```python
from build123d import *

# Parameters (mm, degrees)
F0_W      = 200
F0_H      = 200
F1_DEPTH  = 19.05
F3_D      = 16
F4_W      = 12
F4_H      = 125
F5_DEPTH  = 75
F6_SIZE2  = 75
F6_SIZE   = 50
F9_DEPTH  = 19.05
F11_DEPTH = 500
F12_W     = 50
F12_H     = 5
F13_DEPTH = 90
F14_W     = 5
F14_H     = 80
F15_DEPTH = 70
F16_SIZE2 = 40
F16_SIZE  = 60
F18_DEPTH = 25
F19_W     = 65
F19_H     = 19.05
F20_DEPTH = 25
F21_R     = 10
F22_R     = 6
F23_DEPTH = 25


with BuildPart() as f1:
    # F0 (on Top) → F1 (new body)
    with BuildSketch(Plane.XY):
        Rectangle(F0_W, F0_H)
    extrude(amount=F1_DEPTH)

    # F3 (through all)
    with Locations(Plane.XY.offset(19.05)):
        with Locations((0, 80)):
            Hole(F3_D / 2)

    # F4 (on face) → F5 (join)
    with BuildSketch(Plane(origin=(0, 0, 0), x_dir=(1, 0, 0), z_dir=(0, 0, -1))):
        with Locations((79, 37.5)):
            Rectangle(F4_W, F4_H)
    extrude(amount=F5_DEPTH)

    # F6
    f6_edges = [f1.edges().sort_by_distance(p)[0] for p in [
        (79, 25, -75),
    ]]
    f6_side = f1.faces().sort_by_distance((79, 25, -37.5))[0]
    chamfer(f6_edges, length=F6_SIZE, length2=F6_SIZE2, reference=f6_side)

    # F7: F1 across plane


with BuildPart() as f1_1:
    add(f1.part)
    add(f1.part.mirror(Plane.YZ))

    # F8 (on face) → F9 (join)
    with BuildSketch(Plane.XZ.offset(100)):
        Polygon((100, -85.95), (100, 0), (85, 0), (85, -75), (73, -75), (73, 0), (-73, 0), (-73, -75), (-85, -75), (-85, 0), (-100, 0), (-100, -85.95), align=None)
        Polygon((100, 0), (100, 19.05), (-100, 19.05), (-100, 0), (-85, 0), (-85, -75), (-73, -75), (-73, 0), (73, 0), (73, -75), (85, -75), (85, 0), align=None)
    extrude(amount=F9_DEPTH)

    # F10 (on face) → F11 (cut)
    with BuildSketch(Plane.YZ.offset(85)):
        Polygon((-100, 0), (-100, -21.6502193362), (-68.8245669007, 0), align=None)
    extrude(amount=-F11_DEPTH, mode=Mode.SUBTRACT)

    # F12 (on face) → F13 (join)
    with BuildSketch(Plane(origin=(0, 0, 0), x_dir=(1, 0, 0), z_dir=(0, 0, -1))):
        with Locations((0, -62.5)):
            Rectangle(F12_W, F12_H)
    extrude(amount=F13_DEPTH)

    # F14 (on face) → F15 (join)
    with BuildSketch(Plane(origin=(0, 0, 0), x_dir=(1, 0, 0), z_dir=(0, 0, -1))):
        with Locations((0, -20)):
            Rectangle(F14_W, F14_H)
    extrude(amount=F15_DEPTH)

    # F16
    f16_edges = [f1_1.edges().sort_by_distance(p)[0] for p in [
        (0, -20, -70),
    ]]
    f16_side = f1_1.faces().sort_by_distance((0, 20, -70))[0]
    chamfer(f16_edges, length=F16_SIZE, length2=F16_SIZE2, reference=f16_side)

    # F17 (on face) → F18 (cut)
    with BuildSketch(Plane.YZ.offset(2.5)):
        Polygon((60, 0), (49.0511549105, 0), (60, -8.0538968956), align=None)
    extrude(amount=-F18_DEPTH, mode=Mode.SUBTRACT)

    # F19 (on face) → F20 (join)
    with BuildSketch(Plane(origin=(0, 100, 0), x_dir=(-1, 0, 0), z_dir=(0, 1, 0))):
        with Locations((67.5, 9.525)):
            Rectangle(F19_W, F19_H)
    extrude(amount=F20_DEPTH)

    # F21
    f21_edges = [f1_1.edges().sort_by_distance(p)[0] for p in [
        (-100, 125, 9.525),
        (-35, 125, 9.525),
        (-35, 100, 9.525),
    ]]
    fillet(f21_edges, radius=F21_R)

    # F22 (on face) → F23 (cut)
    with BuildSketch(Plane.XY.offset(19.05)):
        with Locations((-63.2194236771, 108.8713434036)):
            Circle(F22_R)
        with Locations((-68.7925902107, 70.10911874)):
            Circle(F22_R)
        with Locations((-52.5245954176, 34.4871789908)):
            Circle(F22_R)
        with Locations((-19.5804127005, 13.3152383338)):
            Circle(F22_R)
        with Locations((19.5804127005, 13.3152383338)):
            Circle(F22_R)
    extrude(amount=-F23_DEPTH, mode=Mode.SUBTRACT)


solid = f1_1.part
```
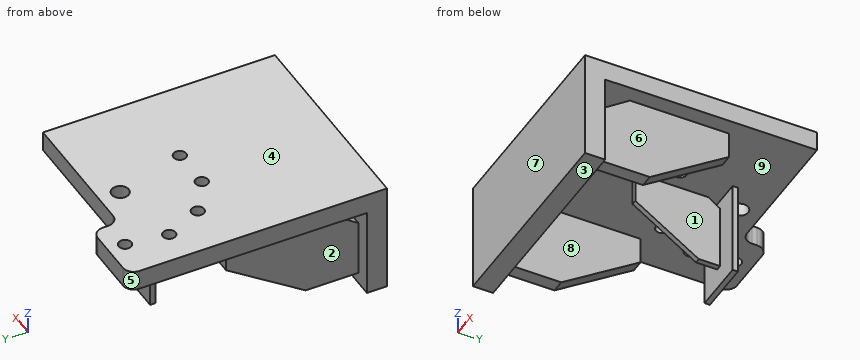
Model file for the job. Use its own axes, mm. Face numbers are marked on the shaded views. A direction names the side the tool comes from. Round coordinates to 2 decimals unless told otherwise and drop trailing zeros. Order: outer loops, then holes, each group sorted by start corner. A loop starts at its lowest first (then second) coordinate and runs counter-clockwise, first axis right, second up. Notation, with made-up numbers: (-8.75, -38.5) -> (11.25, -38.5) arc R14 ccw to (11.25, -15.5) -> close; hole circle Ø10 at (-37, -23.75). An arc over 180 degrees is marked (long way). Use one line per item in the form item = value.
Item 1: Cut at A-A, the plane z = -39.5. Write the cut outline in (x, y), and give its area (3 significant figures).
Returned:
outline = (-100, -119.05) -> (100, -119.05) -> (100, -100) -> (85, -100) -> (85, 3.25) -> (73, 3.25) -> (73, -100) -> (-73, -100) -> (-73, 3.25) -> (-85, 3.25) -> (-85, -100) -> (-100, -100) -> close; (-25, 60) -> (-2.5, 60) -> (-2.5, -5.75) -> (2.5, -5.75) -> (2.5, 60) -> (25, 60) -> (25, 65) -> (-25, 65) -> close
area = 6,870 mm^2
Item 2: Cut at B-B, the plane y = 80. Write the cut outline in (x, z), and give its area (3 significant figures).
Returned:
outline = (-100, 0) -> (-8, 0) -> (-8, 19.05) -> (-100, 19.05) -> close; (8, 0) -> (100, 0) -> (100, 19.05) -> (8, 19.05) -> close
area = 3,510 mm^2
Item 3: Tool access for the marked faces 1, 2, 3, 4 and 5: list every direction of +Z, -Z, +X, -X, +Y, -Y with a clear straight run to the whole face (end or side of a thin tool).
Returned:
face_1 = -Z
face_2 = -Z, -X, +Y
face_3 = -Z, +X, -X, -Y
face_4 = +Z, +X, -X, +Y, -Y
face_5 = +Z, -Z, -X, +Y
Item 4: Drill centre lines: line 1 (X direction, y = -87, z = -47); line 2 (Y direction, x = 3, z = -10); line 3 (Z direction, x = -5, y = 4.5). Where is each one in solid material? Low to high.
Returned:
line_1 = -85 to -73, 73 to 85
line_2 = -119.05 to -100, 60 to 65
line_3 = 0 to 19.05
Item 5: Pull direction X, two halves, no side cores. Call the marked faces 6, 7, 8 and 9: released by +X, released by -X, zero draft, split by the parting line, or undercut.
Returned:
face_6 = released by +X
face_7 = zero draft
face_8 = undercut
face_9 = undercut
Item 6: Cut at D-D, the plane y = -90.5. Write the cut outline in (x, z).
Returned:
outline = (-100, 0) -> (100, 0) -> (100, 19.05) -> (-100, 19.05) -> close; (-85, -75) -> (-73, -75) -> (-73, -15.05) -> (-85, -15.05) -> close; (73, -75) -> (85, -75) -> (85, -15.05) -> (73, -15.05) -> close
Item 7: Flat gauge pins, fed straight in: pin 1 Ø1 at (y, z) = (51.5, -28.5) entering from +X; pin 2 Ø1 at (y, z) = (-47.5, -23.5) entering from -X; pin 3 Ø15 at (x, y) = (-39, -110.5) entering from -Z. Where does each tip first touch, or does it go through?
Returned:
pin_1 = 2.5
pin_2 = -85
pin_3 = -85.95
Item 8: Cut at C-C, the plane x = -78. Write the cut outline in (y, z).
Returned:
outline = (-119.05, -85.95) -> (-100, -85.95) -> (-100, -75) -> (-50, -75) -> (25, -25) -> (25, 0) -> (125, 0) -> (125, 19.05) -> (-119.05, 19.05) -> close; hole (-100, -21.65) -> (-68.82, 0) -> (-100, 0) -> close
